Build history of the part. All positions in model axes, mm. Face numbers are marked on the shaded views. A direction names the side the tool comes from. Round coordinates to 2 decimals unless told otherwise and drop trailing zeros. Write each loop counter-clockwise with the first axis right and the second up, starting at its lowest first coordinate (ties: lowest second). Pieces come first, ordered by that corner, then holes. Notation, with made-up numbers: M 75,-35.75 L 117,-35.75 A16 ccw 117,-27.75 Z; hole C -11,62.5 d3. An arc over 180 degrees is marked long. Use a Markdown table: item, result.
from build123d import *

# Parameters (mm, degrees)
BOSS_EXTRUDE5_DEPTH     = 20.32
BOSS_EXTRUDE6_DEPTH     = 2.54
SKETCH3_R               = 1.905
CUT_EXTRUDE3_DEPTH      = 25.13
CUT_EXTRUDE3_DEPTH_BACK = 1
FILLET3_R               = 2.54


with BuildPart() as part:
    # Sketch2 → Boss-Extrude5 (new body)
    with BuildSketch(Plane.XY):
        with BuildLine():
            Line((19.702242383, 36.423556552), (19.702242383, 0))
            Line((19.702242383, 0), (24.13, 0))
            Line((24.13, 0), (24.13, 37.9095))
            ThreePointArc((24.13, 37.9095), (7.9375, 54.102), (24.13, 70.2945))
            Line((24.13, 70.2945), (24.13, 82.55))
            Line((24.13, 82.55), (19.702242383, 82.55))
            Line((19.702242383, 82.55), (19.702242383, 71.780443448))
            ThreePointArc((19.702242383, 71.780443448), (5.9055, 54.102), (19.702242383, 36.423556552))
        make_face()
    extrude(amount=BOSS_EXTRUDE5_DEPTH)

    # Sketch2<7> → Boss-Extrude6 (add)
    with BuildSketch(Plane.XY):
        with BuildLine():
            Line((0, 82.55), (0, 0))
            Line((0, 0), (19.702242383, 0))
            Line((19.702242383, 0), (19.702242383, 36.423556552))
            ThreePointArc((19.702242383, 36.423556552), (5.9055, 54.102), (19.702242383, 71.780443448))
            Line((19.702242383, 71.780443448), (19.702242383, 82.55))
            Line((19.702242383, 82.55), (0, 82.55))
        make_face()
    extrude(amount=BOSS_EXTRUDE6_DEPTH)

    # Sketch3 → Cut-Extrude3 (cut, two sides)
    with BuildSketch(Plane(origin=(0, 0, 0), x_dir=(0, 0, -1), z_dir=(1, 0, 0))) as cut_extrude3_sk:
        with Locations((-12.7, 18.430889618)):
            Circle(SKETCH3_R)
        with Locations((-12.7, 76.946110382)):
            Circle(SKETCH3_R)
    extrude(amount=CUT_EXTRUDE3_DEPTH, mode=Mode.SUBTRACT)
    extrude(cut_extrude3_sk.sketch, amount=-CUT_EXTRUDE3_DEPTH_BACK, mode=Mode.SUBTRACT)

    # Fillet3
    fillet3_edges = [part.edges().sort_by_distance(p)[0] for p in [
        (5.9055, 54.102, 2.54),
        (19.702242383, 77.165221724, 2.54),
        (19.702242383, 18.211778276, 2.54),
    ]]
    fillet(fillet3_edges, radius=FILLET3_R)


solid = part.part
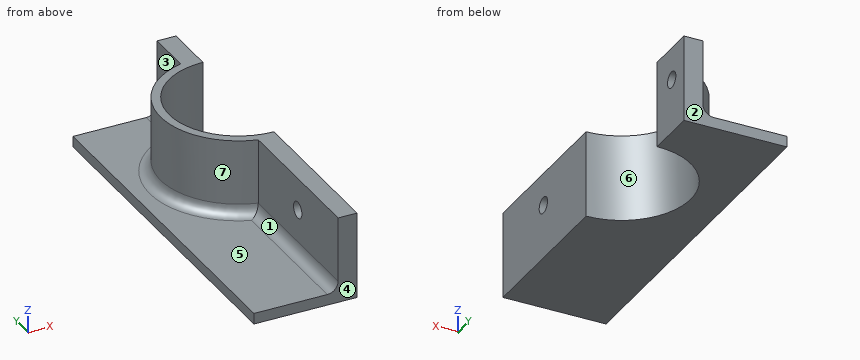
Q1. Cut at A-A on z = 12.7. Count the separate pieces of the cut face and the enclosed holes in it, and give its area (3 significant figures).
Response values:
| item | result |
|---|---|
| separate pieces | 3 |
| enclosed holes | 0 |
| area | 282 mm2 |
Q2. Drill centre lines: L1, parallel to Y at x = 21.65, z = 12.7; L2, parallel to Y at x = 22.15, z = 12.7; L3, parallel to Z at x = 3.5, y = 5.5. Where is each one in solid material? Low to high.
Response values:
| item | result |
|---|---|
| L1 | y = 0 to 16.53, 20.34 to 38.1, 70.1 to 75.04, 78.85 to 82.55 |
| L2 | y = 0 to 16.53, 20.34 to 38.03, 70.17 to 75.04, 78.85 to 82.55 |
| L3 | z = 0 to 2.54 |
Q3. Which spindle directions (+Z, -Z, +X, -X, +Y, -Y) get a long thin tool onto all of the face, cutting with end or side? Do the marked faces 1, 2 and 3. Say none if no direction does.
Response values:
| item | result |
|---|---|
| face 1 | +Z, -X, -Y |
| face 2 | +Z, -Z, +X, -X, +Y |
| face 3 | +Z, -X, +Y |
Q4. Cut at C-C on y = 19.5. Give the cut face in (x, z), and give its area (3 significant figures).
Response values:
| item | result |
|---|---|
| outline | M 0,0 L 24.13,0 L 24.13,11.12 L 19.7,11.12 L 19.7,5.08 A2.54 cw 17.16,2.54 L 0,2.54 Z; M 19.7,14.28 L 24.13,14.28 L 24.13,20.32 L 19.7,20.32 Z |
| area | 127 mm2 |
Q5. Drop flat-ended pins along their axis: P1, Ø3, axis at y = 18.43, z = 12.7, coming from the -X side; P2, Ø2, axis at x = 15, z = 11, coming from the +Y side; P3, Ø12, axis at y = 16, z = 16, coming from the -X side; P4, Ø5, axis at x = 7, y = 36.5, coming from the +Z side. Give the stop position or say it passes through.
Response values:
| item | result |
|---|---|
| P1 | passes through |
| P2 | stops at y = 70.41 |
| P3 | stops at x = 19.7 |
| P4 | stops at z = 2.54 |
Q6. Cut at B-B on x = 22.25. Give the cut face in (y, z) (3 decimals), and give its area (3 significant figures).
Response values:
| item | result |
|---|---|
| outline | M 0,0 L 38.019,0 L 38.019,20.32 L 0,20.32 Z; M 70.185,0 L 82.55,0 L 82.55,20.32 L 70.185,20.32 Z; hole C 18.431,12.7 d3.81; hole C 76.946,12.7 d3.81 |
| area | 1,000 mm2 |
Q7. Two-plate mould, pull along Y, no slides. Class the marked faces 4, 5, 6 and 7: +Y half, -Y half, draft (parallel to the pull), parting line (faces both ways), or undercut.
Response values:
| item | result |
|---|---|
| face 4 | -Y half |
| face 5 | draft |
| face 6 | undercut |
| face 7 | parting line |
